from build123d import *

# Parameters (mm, degrees)
BOSS_EXTRUDE1_DEPTH = 10
CUT_EXTRUDE5_REACH  = 103.397
SKETCH9_R           = 1.5
FILLET10_R          = 3
FILLET11_R          = 3
FILLET12_R          = 3
FILLET13_R          = 7.5
FILLET14_R          = 15
FILLET16_R          = 15
FILLET18_R          = 15
FILLET19_R          = 7.5
FILLET22_R          = 3
FILLET23_R          = 3
FILLET24_R          = 15
FILLET25_R          = 3
FILLET26_R          = 3
FILLET27_R          = 3
FILLET28_R          = 3
FILLET29_R          = 3
FILLET30_R          = 3
FILLET31_R          = 3
SKETCH11_R          = 1.5
CUT_EXTRUDE6_DEPTH  = 7.5
FILLET32_R          = 7.5
FILLET33_R          = 5
FILLET34_R          = 7.5
FILLET36_R          = 5


with BuildPart() as part:
    # Sketch1 → Boss-Extrude1 (new body)
    with BuildSketch(Plane(origin=(0, 0, 0), x_dir=(1, 0, 0), z_dir=(0, 1, 0))):
        with BuildLine():
            Line((0, -12.5), (0, -60))
            Line((0, -60), (22.5, -60))
            Line((22.5, -60), (81.125, -22.5))
            Line((81.125, -22.5), (81.125, 0))
            Line((81.125, 0), (75.125, 0))
            ThreePointArc((75.125, 0), (62.625, -12.5), (50.125, 0))
            Line((50.125, 0), (44.125, 0))
            Line((44.125, 0), (44.125, -12.5))
            Line((44.125, -12.5), (0, -12.5))
        make_face()
        Polygon((39.125, -17.5), (45.538841531, -34.595428821), (22.483333333, -50), (5, -50), (5, -17.5), align=None, mode=Mode.SUBTRACT)
        Polygon((71.125, -17.5), (49.69624181, -31.817655806), (44.125, -17.5), align=None, mode=Mode.SUBTRACT)
    boss_extrude1 = extrude(amount=BOSS_EXTRUDE1_DEPTH)

    # Mirror1: Boss-Extrude1 across plane
    add(boss_extrude1.mirror(Plane(origin=(0, 10, 0), x_dir=(0, 0, 1), z_dir=(-1, 0, 0))))

    # Sketch9 → Cut-Extrude5 (cut, up to next)
    with BuildSketch(Plane.XY.offset(60), mode=Mode.PRIVATE) as cut_extrude5_sk1:
        with Locations((-17.75, 5)):
            Circle(SKETCH9_R)
    cut_extrude5_tool1 = extrude(cut_extrude5_sk1.sketch, amount=-CUT_EXTRUDE5_REACH, mode=Mode.PRIVATE) & part.part
    cut_extrude5 = cut_extrude5_tool1.solids().sort_by_distance((-17.75, 5, 60))[0]
    add(cut_extrude5, mode=Mode.SUBTRACT)

    # Mirror2: Cut-Extrude5 across plane
    add(cut_extrude5.mirror(Plane(origin=(0, 0, 0), x_dir=(0, 0, 1), z_dir=(1, 0, 0))), mode=Mode.SUBTRACT)

    # Fillet10
    fillet10_edges = [part.edges().sort_by_distance(p)[0] for p in [
        (71.125, 5, 17.5),
    ]]
    fillet(fillet10_edges, radius=FILLET10_R)

    # Fillet11
    fillet11_edges = [part.edges().sort_by_distance(p)[0] for p in [
        (44.125, 5, 17.5),
    ]]
    fillet(fillet11_edges, radius=FILLET11_R)

    # Fillet12
    fillet12_edges = [part.edges().sort_by_distance(p)[0] for p in [
        (49.69624181, 5, 31.817655806),
    ]]
    fillet(fillet12_edges, radius=FILLET12_R)

    # Fillet13
    fillet13_edges = [part.edges().sort_by_distance(p)[0] for p in [
        (39.125, 5, 17.5),
    ]]
    fillet(fillet13_edges, radius=FILLET13_R)

    # Fillet14
    fillet14_edges = [part.edges().sort_by_distance(p)[0] for p in [
        (45.538841531, 5, 34.595428821),
    ]]
    fillet(fillet14_edges, radius=FILLET14_R)

    # Fillet16
    fillet16_edges = [part.edges().sort_by_distance(p)[0] for p in [
        (5, 5, 17.5),
    ]]
    fillet(fillet16_edges, radius=FILLET16_R)

    # Fillet18
    fillet18_edges = [part.edges().sort_by_distance(p)[0] for p in [
        (-5, 5, 17.5),
    ]]
    fillet(fillet18_edges, radius=FILLET18_R)

    # Fillet19
    fillet19_edges = [part.edges().sort_by_distance(p)[0] for p in [
        (-39.125, 5, 17.5),
    ]]
    fillet(fillet19_edges, radius=FILLET19_R)

    # Fillet22
    fillet22_edges = [part.edges().sort_by_distance(p)[0] for p in [
        (44.125, 5, 12.5),
    ]]
    fillet(fillet22_edges, radius=FILLET22_R)

    # Fillet23
    fillet23_edges = [part.edges().sort_by_distance(p)[0] for p in [
        (-44.125, 5, 12.5),
    ]]
    fillet(fillet23_edges, radius=FILLET23_R)

    # Fillet24
    fillet24_edges = [part.edges().sort_by_distance(p)[0] for p in [
        (-45.538841531, 5, 34.595428821),
    ]]
    fillet(fillet24_edges, radius=FILLET24_R)

    # Fillet25
    fillet25_edges = [part.edges().sort_by_distance(p)[0] for p in [
        (-44.125, 5, 17.5),
    ]]
    fillet(fillet25_edges, radius=FILLET25_R)

    # Fillet26
    fillet26_edges = [part.edges().sort_by_distance(p)[0] for p in [
        (-49.69624181, 5, 31.817655806),
    ]]
    fillet(fillet26_edges, radius=FILLET26_R)

    # Fillet27
    fillet27_edges = [part.edges().sort_by_distance(p)[0] for p in [
        (-71.125, 5, 17.5),
    ]]
    fillet(fillet27_edges, radius=FILLET27_R)

    # Fillet28
    fillet28_edges = [part.edges().sort_by_distance(p)[0] for p in [
        (22.5, 5, 60),
    ]]
    fillet(fillet28_edges, radius=FILLET28_R)

    # Fillet29
    fillet29_edges = [part.edges().sort_by_distance(p)[0] for p in [
        (-22.5, 5, 60),
    ]]
    fillet(fillet29_edges, radius=FILLET29_R)

    # Fillet30
    fillet30_edges = [part.edges().sort_by_distance(p)[0] for p in [
        (81.125, 5, 22.5),
    ]]
    fillet(fillet30_edges, radius=FILLET30_R)

    # Fillet31
    fillet31_edges = [part.edges().sort_by_distance(p)[0] for p in [
        (-81.125, 5, 22.5),
    ]]
    fillet(fillet31_edges, radius=FILLET31_R)

    # Sketch11 → Cut-Extrude6 (cut)
    with BuildSketch(Plane(origin=(0, 0, 0), x_dir=(-1, 0, 0), z_dir=(0, 0, -1))):
        with Locations((-78.125, 5)):
            Circle(SKETCH11_R)
        with Locations((-47.125, 5)):
            Circle(SKETCH11_R)
    cut_extrude6 = extrude(amount=-CUT_EXTRUDE6_DEPTH, mode=Mode.SUBTRACT)

    # Mirror3: Cut-Extrude6 across plane
    add(cut_extrude6.mirror(Plane(origin=(0, 0, 0), x_dir=(0, 0, 1), z_dir=(1, 0, 0))), mode=Mode.SUBTRACT)

    # Fillet32
    fillet32_edges = [part.edges().sort_by_distance(p)[0] for p in [
        (5, 5, 50),
    ]]
    fillet(fillet32_edges, radius=FILLET32_R)

    # Fillet33
    fillet33_edges = [part.edges().sort_by_distance(p)[0] for p in [
        (22.483333333, 5, 50),
    ]]
    fillet(fillet33_edges, radius=FILLET33_R)

    # Fillet34
    fillet34_edges = [part.edges().sort_by_distance(p)[0] for p in [
        (-5, 5, 50),
    ]]
    fillet(fillet34_edges, radius=FILLET34_R)

    # Fillet36
    fillet36_edges = [part.edges().sort_by_distance(p)[0] for p in [
        (-22.483333333, 5, 50),
    ]]
    fillet(fillet36_edges, radius=FILLET36_R)


solid = part.part
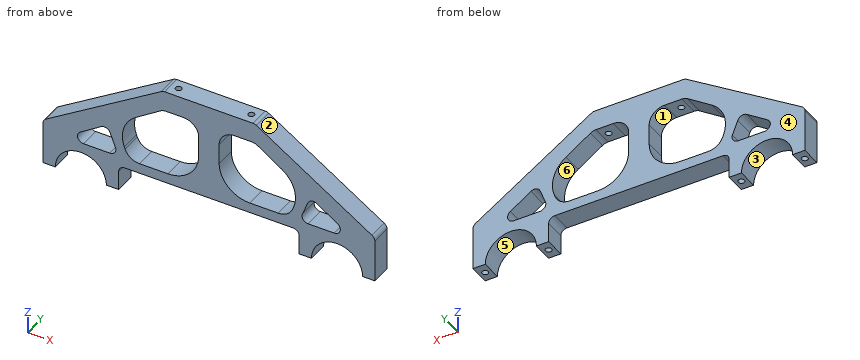
CAD build for the part. Positions are in the model's coordinates, mm. Face numbers are marked on the shaded views. A direction names the side the tool comes from. Give positions to 0.01 mm unless a question says otherwise; leave off trailing zeros. Write each loop counter-clockwise with the first axis right and the second up, starting at its lowest first coordinate (ties: lowest second). Pieces come first, ordered by that corner, then holes. Notation, with made-up numbers: (-31.5, -15.5) -> (-21.5, -15.5) arc R16 ccw to (-21.5, -9.5) -> close; hole circle Ø5 at (-5, -30). An arc over 180 degrees is marked (long way). Return JSON: item names as keys, results as strings.
Item 1: Tool access for the marked faces 5 and 6: list every direction of +Z, -Z, +X, -X, +Y, -Y with a clear straight run to the whole face (end or side of a thin tool).
Answer below:
{"face 5": "-Z, +Y, -Y", "face 6": "+Y, -Y"}
Item 2: Two-plate mould, pull along Z, no slides. Class the marked faces 1, 2, 3 and 4: +Z half, -Z half, draft (parallel to the pull), parting line (faces both ways), or undercut.
Answer below:
{"face 1": "undercut", "face 2": "+Z half", "face 3": "-Z half", "face 4": "draft"}
Item 3: Band-saw the part on A-A (x = -57.5). List the corners of the cut face in (y, z), then the cut area to 3 significant figures.
Answer below:
{"outline": "(0, 11.4) -> (10, 11.4) -> (10, 17.5) -> (0, 17.5) -> close; (0, 26.6) -> (10, 26.6) -> (10, 37.61) -> (0, 37.61) -> close", "area": "171 mm2"}
Item 4: Band-saw the part on D-D (x = 17.75). List the corners of the cut face in (y, z).
Answer below:
{"outline": "(0, 12.5) -> (10, 12.5) -> (10, 17.67) -> (0, 17.67) -> close; (0, 50) -> (3.5, 50) -> (3.5, 60) -> (0, 60) -> close; (6.5, 50) -> (10, 50) -> (10, 60) -> (6.5, 60) -> close"}
Item 5: Drill centre lines: probe 1 along X at (y, z) = (5.5, 19.5) (3 decimals); probe 2 along X at (y, z) = (3.75, 21); probe 3 along X at (y, z) = (6, 54). Where is each one in solid material? Low to high.
Answer below:
{"probe 1": "x = -81.125 to -64.063, -45.683 to -39.027, -12.517 to 12.517, 39.027 to 45.683, 64.063 to 81.125", "probe 2": "x = -81.12 to -64.19, -45.55 to -40.27, -10.37 to 10.37, 40.27 to 45.55, 64.19 to 81.12", "probe 3": "x = -31.88 to -18.87, -16.63 to 16.63, 18.87 to 31.88"}
Item 6: Band-saw the part on B-B (y = 5). Give the number of separate pieces and of enclosed holes in the cut face, then the cut area to 3 significant figures.
Answer below:
{"separate pieces": "1", "enclosed holes": "2", "area": "3,480 mm2"}
Item 7: Band-saw the part on C-C (z = 37). List the corners of the cut face in (x, y).
Answer below:
{"outline": "(-58.46, 0) -> (-39.83, 0) -> (-39.83, 10) -> (-58.46, 10) -> close; (-5, 0) -> (5, 0) -> (5, 10) -> (-5, 10) -> close; (39.83, 0) -> (58.46, 0) -> (58.46, 10) -> (39.83, 10) -> close"}
Item 8: Drop flat-ended pins along their axis: pin 1 (1.8 mm diameter, centred on x = 47.125, y = 5, fed in from +Z); pin 2 (1.5 mm diameter, centred on x = -47, y = 5.5, fed in from -Z); pin 3 (5 mm diameter, centred on x = 78.125, y = 5, fed in from +Z). Give the stop position or say it passes through.
Answer below:
{"pin 1": "stops at z = 44.82", "pin 2": "stops at z = 7.5", "pin 3": "stops at z = 26.02"}
